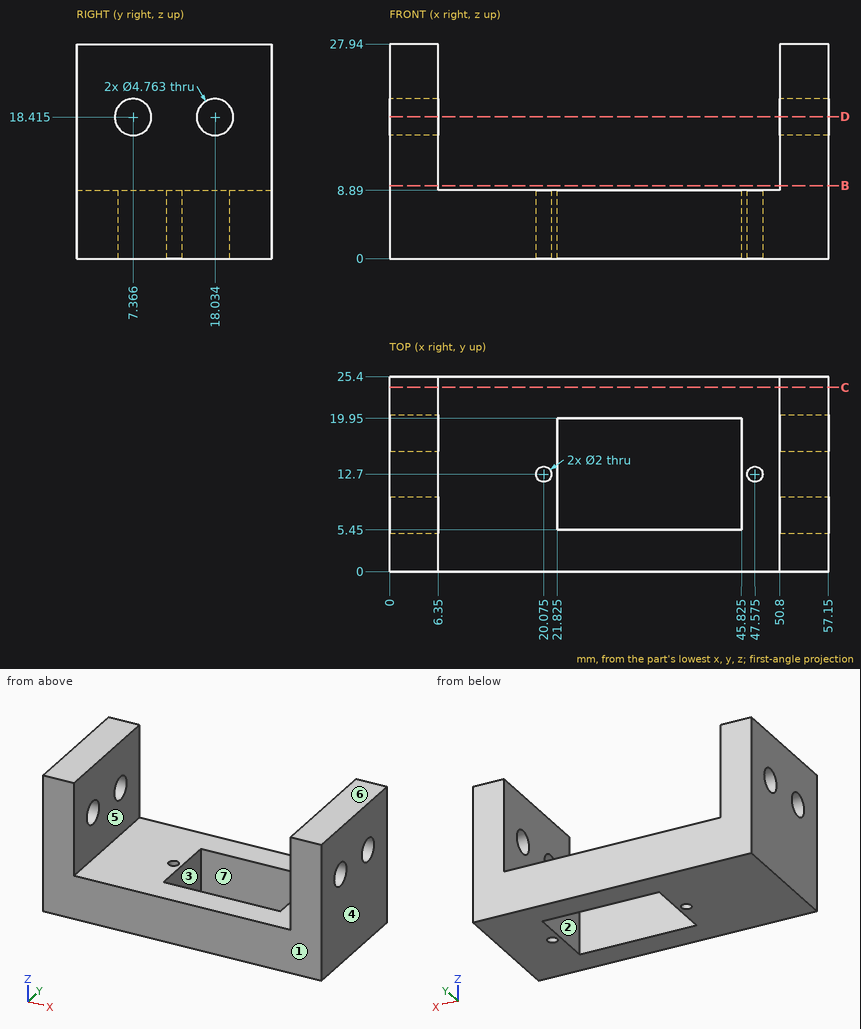
Check sheet for the drawn part. Datum: minimum x, y, z corner. Units: mm. A direction names the side the tool comes from. Round coordinates to 2 decimals unless told otherwise and drop trailing zeros. Loops run counter-clockwise (first coordinate to the right, second up) from the corner with the lowest first, then second, coordinate; pieces in that order, holes last. Notation, with made-up numbers: M 68.25,-31.5 L 78.25,-31.5 A31 cw 78.25,4.5 Z; hole C 73,-19.75 d3. An arc over 180 degrees is marked long. One line per question, with ' | ' between items. Start each with the question number.
Item 1: Section check D-D (z = 18.5). State how many separate pieces and enclosed holes the cut face has, and give its area (3 significant figures).
Item 2: Set-up check for the marked faces 5, 6 and 7: record each of +Z, -Z, +X, -X, +Y, -Y from which the full face is reachable in a straight line by a thin tool's end or side.
Item 3: Section check C-C (y = 24). Record the boundary of the cut face in (x, z).
Item 4: Scan lines: probe 1 along X at (y, z) = (5.5, 15.25); probe 2 along Z at (x, y) = (54.5, 7.25); probe 3 along Z at (x, y) = (41, 3.25). Record each from-to range of solid material in increasing order.
Item 5: Section check B-B (z = 9.5). Record the boundary of the cut face in (x, y).
Item 6: Release check for a two-part mould opening along Y. For the marked faces 1, 2, 3 and 4 record: released by +Y, released by -Y, zero draft, split by the parting line, or undercut.
Worked out:
1) separate pieces: 6 | enclosed holes: 0 | area: 202 mm^2
2) face 5: +Z, +Y, -Y | face 6: +Z, +X, -X, +Y, -Y | face 7: +Z, -Z
3) outline: M 0,0 L 57.15,0 L 57.15,27.94 L 50.8,27.94 L 50.8,8.89 L 6.35,8.89 L 6.35,27.94 L 0,27.94 Z
4) probe 1: 0 to 6.35, 50.8 to 57.15 | probe 2: 0 to 16.04, 20.79 to 27.94 | probe 3: 0 to 8.89
5) outline: M 0,0 L 6.35,0 L 6.35,25.4 L 0,25.4 Z; M 50.8,0 L 57.15,0 L 57.15,25.4 L 50.8,25.4 Z
6) face 1: released by -Y | face 2: undercut | face 3: undercut | face 4: zero draft
